from build123d import *

# Parameters (mm, degrees)
SKETCH_2_R          = 8.5
EXTRUDE_1_DEPTH     = 4
SKETCH_3_RX         = 25
SKETCH_3_RY         = 7.848678542
CUT_EXTRUDE_1_DEPTH = 10


with BuildPart() as part:
    # 草图2 → 凸台-拉伸1 (new body)
    with BuildSketch(Plane(origin=(0, 0, 0), x_dir=(0, 0, -1), z_dir=(1, 0, 0))):
        with BuildLine():
            ThreePointArc((38.448053475, 47.999970666), (48.038029113, 50.902904709), (56.98733583, 46.396845666))
            Line((56.98733583, 46.396845666), (90.11233583, 8.94375))
            ThreePointArc((90.11233583, 8.94375), (92.308343207, -5.545690895), (80, -13.5))
            Line((80, -13.5), (0, -13.5))
            ThreePointArc((0, -13.5), (-12.74034561, -4.464705337), (-8.426946525, 10.546875))
            Line((-8.426946525, 10.546875), (38.448053475, 47.999970666))
        make_face()
        with Locations((80, 0)):
            Circle(SKETCH_2_R, mode=Mode.SUBTRACT)
        with Locations((46.875, 37.453095666)):
            Circle(SKETCH_2_R, mode=Mode.SUBTRACT)
        Circle(SKETCH_2_R, mode=Mode.SUBTRACT)
    extrude(amount=EXTRUDE_1_DEPTH)

    # 草图3 → 切除-拉伸1 (cut)
    with BuildSketch(Plane(origin=(4, 0, 0), x_dir=(0, 0, -1), z_dir=(1, 0, 0))):
        with Locations((40, 0)):
            Ellipse(SKETCH_3_RX, SKETCH_3_RY)
    extrude(amount=-CUT_EXTRUDE_1_DEPTH, mode=Mode.SUBTRACT)


solid = part.part
For this review, take the finished solid that the model builds, in its own axes (mm). Give positions to 0.01 mm unless a question says otherwise; leave off trailing zeros. Loops run counter-clockwise (first coordinate to the right, second up) from the corner with the lowest first, then second, coordinate; pieces in that order, holes last. Notation, with made-up numbers: M 55,79 L 98,79 A13 ccw 98,91 Z; hole C -34.75,-9.5 d9. An arc over 180 degrees is marked long. Answer as a JSON object with one key per item and string values. Group by question number.
Q1. Insertion check: P1, Ø6, axis at y = 2, z = -61.5, coming from the -X side. The pin has a flat end and moves straight along its axis. Give the tip position at first contact, or say it passes through.
Q2. Mouldability with a two-part tool opening along Y and no side actions: class faces 1 (the cylindrical face through (1.97, 0.37, -71.51)), 2 (the cylindrical face through (1.972, -5.347, -92.396)), 3 (the flat face through (1.97, 27.93, -73.32)) as +Y half, -Y half, draft (parallel to the pull), parting line (faces both ways), or undercut.
Q3. Add section B-B on z = -5.5. Give the boundary of the cut face in (x, y).
Q4. Add section C-C on y = 0. Give the number of separate pieces and of enclosed holes in the cut face, and give its area (3 significant figures).
Q5. For probe 1 along Z at (x, y) = (0.35, -1); probe 2 along Y at (x, z) = (1.8, -45); probe 3 along Y at (x, z) = (1.35, -23), list the stretches that pass through material, from the lowest coordinate up. Write a range as [from, to].
Q6. Add section A-A on y = 41. Give the boundary of the cut face in (x, z).
Checked values:
{
 "1": {"P1": "x = 0"},
 "2": {"face 1": "undercut", "face 2": "parting line", "face 3": "+Y half"},
 "3": {"outline": "M 0,-13.5 L 4,-13.5 L 4,-6.48 L 0,-6.48 Z; M 0,6.48 L 4,6.48 L 4,21.67 L 0,21.67 Z"},
 "4": {"separate pieces": "4", "enclosed holes": "0", "area": "92.0 mm²"},
 "5": {"probe 1": "[-93.46, -88.44], [-71.56, -64.8], [-15.2, -8.44], [8.44, 13.46]", "probe 2": "[-13.5, -7.69], [7.69, 29.16], [45.74, 50.82]", "probe 3": "[-13.5, -5.75], [5.75, 35.66]"},
 "6": {"outline": "M 0,-61.76 L 4,-61.76 L 4,-54.6 L 0,-54.6 Z; M 0,-39.15 L 4,-39.15 L 4,-29.69 L 0,-29.69 Z"}
}
